from build123d import *

# Parameters (mm, degrees)
SKETCH1_R           = 75
BOSS_EXTRUDE1_DEPTH = 10
SKETCH3_R           = 40
BOSS_EXTRUDE2_DEPTH = 10
SKETCH4_R           = 35
CUT_EXTRUDE1_DEPTH  = 20
SKETCH5_R           = 5
CUT_EXTRUDE2_DEPTH  = 20


with BuildPart() as part:
    # Sketch1 → Boss-Extrude1 (new body)
    with BuildSketch(Plane.XY):
        Circle(SKETCH1_R)
    extrude(amount=BOSS_EXTRUDE1_DEPTH)

    # Sketch2 → Revolve1 (revolve)
    with BuildSketch(Plane(origin=(0, 0, 0), x_dir=(0, 0, -1), z_dir=(1, 0, 0)), mode=Mode.PRIVATE) as revolve1_sk:
        with BuildLine():
            Line((-10, 45), (-20, 45))
            ThreePointArc((-20, 45), (-27.117468017, 34.188611699), (-39.364916731, 30))
            Line((-39.364916731, 30), (-85, 30))
            Line((-85, 30), (-85, 0))
            Line((-85, 0), (-10, 0))
            Line((-10, 0), (-10, 45))
        make_face()
    revolve(revolve1_sk.sketch.rotate(Axis((0, 0, 1000), (0, 0, -1)), 90), axis=Axis((0, 0, 1000), (0, 0, -1)))

    # Sketch3 → Boss-Extrude2 (add)
    with BuildSketch(Plane(origin=(0, 0, 0), x_dir=(-1, 0, 0), z_dir=(0, 0, -1))):
        Circle(SKETCH3_R)
    extrude(amount=BOSS_EXTRUDE2_DEPTH)

    # Sketch4 → Cut-Extrude1 (cut)
    with BuildSketch(Plane(origin=(0, 0, -10), x_dir=(-1, 0, 0), z_dir=(0, 0, -1))):
        Circle(SKETCH4_R)
    extrude(amount=-CUT_EXTRUDE1_DEPTH, mode=Mode.SUBTRACT)

    # Sketch5 → Cut-Extrude2 (cut)
    with BuildSketch(Plane.XY.offset(10)):
        with Locations((60, 0)):
            Circle(SKETCH5_R)
        with Locations((30, -51.961524227)):
            Circle(SKETCH5_R)
        with Locations((-30, -51.961524227)):
            Circle(SKETCH5_R)
        with Locations((-60, 0)):
            Circle(SKETCH5_R)
        with Locations((-30, 51.961524227)):
            Circle(SKETCH5_R)
        with Locations((30, 51.961524227)):
            Circle(SKETCH5_R)
    extrude(amount=-CUT_EXTRUDE2_DEPTH, mode=Mode.SUBTRACT)


solid = part.part
Verification items for the finished model (mm, model axes). A direction names the side the tool comes from. Give positions to 0.01 mm unless a question says otherwise; leave off trailing zeros. Write each loop counter-clockwise with the first axis right and the second up, starting at its lowest first coordinate (ties: lowest second). Pieces come first, ordered by that corner, then holes. Notation, with made-up numbers: (48.5, -37) -> (98.5, -37) arc R24 cw to (98.5, 0) -> close; hole circle Ø8 at (7.5, 30). An arc over 180 degrees is marked (long way). Use CSV: the item, a comma, the result in double quotes.
(1) Set-up check for faces 1 (the flat face through (32, -32, 10)), 2 (the flat face through (0, 0, 10)), 3 (the flat face through (0, 0, 85)): record each of +Z, -Z, +X, -X, +Y, -Y from which the full face is reachable in a straight line by a thin tool's end or side.
Derived:
face 1,"+Z"
face 2,"-Z"
face 3,"+Z, +X, -X, +Y, -Y"
(2) Sectioned sample at B-B (y = -54). Record the cut outline in (x, z), plus the area to 3 significant figures.
Derived:
outline,"(-52.05, 0) -> (-34.57, 0) -> (-34.57, 10) -> (-52.05, 10) -> close; (-25.43, 0) -> (25.43, 0) -> (25.43, 10) -> (-25.43, 10) -> close; (34.57, 0) -> (52.05, 0) -> (52.05, 10) -> (34.57, 10) -> close"
area,"858 mm^2"
(3) Material ranges on L1, parallel to Y at x = 30, z = 7.5; L2, parallel to X at y = 1.5, z = 5 (3 decimals); L3, parallel to Z at x = 23, y = 69.5, recorded low to high.
Derived:
L1,"y = -68.74 to -56.96, -46.96 to -18.03, 18.03 to 46.96, 56.96 to 68.74"
L2,"x = -74.985 to -64.77, -55.23 to -34.968, 34.968 to 55.23, 64.77 to 74.985"
L3,"z = 0 to 10"
(4) Sectioned sample at C-C (x = 0). Record the cut outline in (y, z).
Derived:
outline,"(-75, 0) -> (-40, 0) -> (-40, -10) -> (-35, -10) -> (-35, 10) -> (35, 10) -> (35, -10) -> (40, -10) -> (40, 0) -> (75, 0) -> (75, 10) -> (45, 10) -> (45, 20) arc R20 cw to (30, 39.36) -> (30, 85) -> (-30, 85) -> (-30, 39.36) arc R20 cw to (-45, 20) -> (-45, 10) -> (-75, 10) -> close"
(5) Release check for a two-part mould opening along X. For faces 4 (the flat face through (0.2, -35.4, -10)), 5 (the cylindrical face through (-9.764, 74.362, 4.93)), 6 (the cylindrical face through (-65, 0, 5)) record: +X half, -X half, draft (parallel to the pull), parting line (faces both ways), or undercut.
Derived:
face 4,"draft"
face 5,"parting line"
face 6,"undercut"
(6) Sectioned sample at A-A (x = 60). Record the cut outline in (y, z), plus the area to 3 significant figures.
Derived:
outline,"(-45, 0) -> (-5, 0) -> (-5, 10) -> (-45, 10) -> close; (5, 0) -> (45, 0) -> (45, 10) -> (5, 10) -> close"
area,"800 mm^2"
(7) Sectioned sample at D-D (z = 46). Record the cut outline in (x, y).
Derived:
outline,"circle Ø60 at (0, 0)"
(8) Go/stop test with flat-tipped pins: pin 1 (11.5 mm diameter, centred on x = 30, y = 51.96, fed in from -Z); pin 2 (9 mm diameter, centred on x = -60, y = 0, fed in from +Z); pin 3 (21 mm diameter, centred on x = 7, y = 5.5, fed in from -Z); pin 4 (5 mm diameter, centred on x = -35, z = 15.5, fed in from +Y). Record where each tip stops, or that it passes through.
Derived:
pin 1,"stops at z = 0"
pin 2,"passes through"
pin 3,"stops at z = 10"
pin 4,"stops at y = 31.12"
